Drawing for the job (mm, zero at the part's lowest x, y, z). Coordinates: 2 decimals unless noted, no trailing zeros. Order: outer loops, then holes, each group sorted by start corner. A loop starts at its lowest first (then second) coordinate and runs counter-clockwise, first axis right, second up. Notation, with made-up numbers: (-38.5, -11) -> (-6.5, -11) arc R20 ccw to (-6.5, 18) -> close; hole circle Ø6 at (19, 71.5). An arc over 180 degrees is marked (long way). Write each question's results on one line, items separated by ' | '.
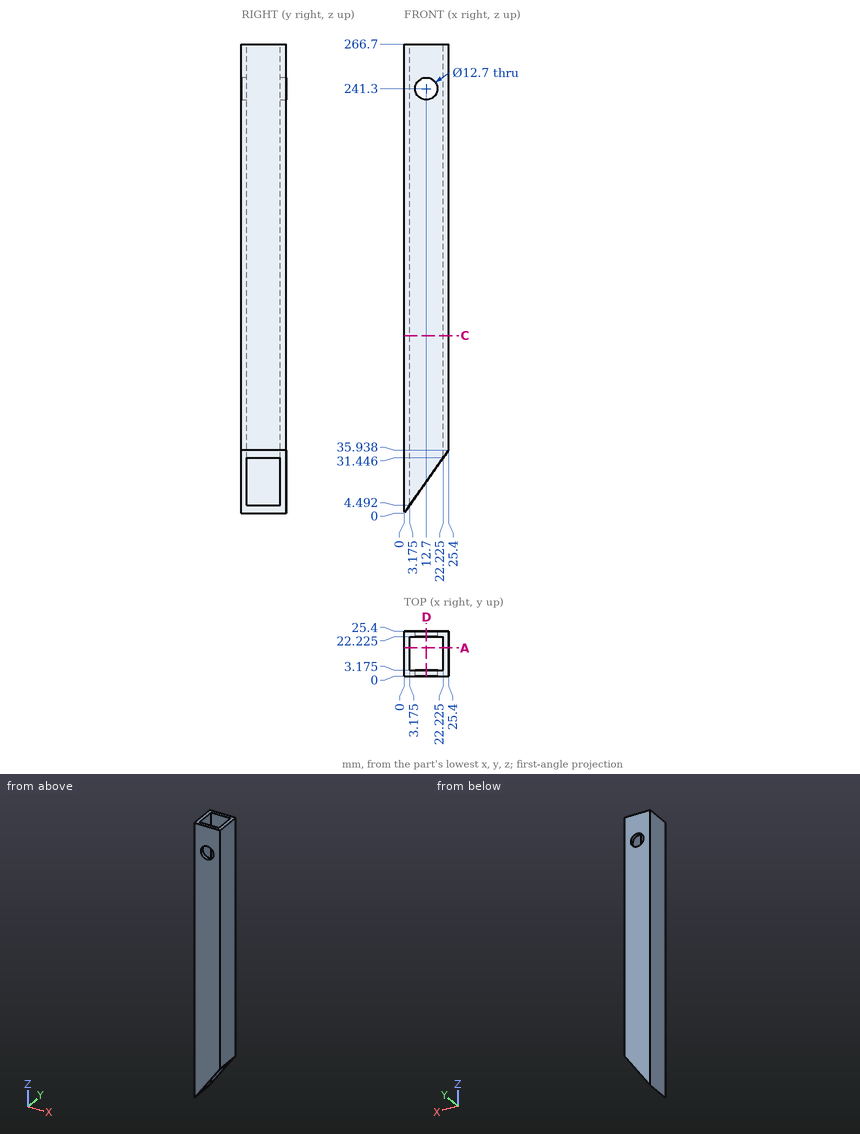
Item 1: Slice it at D-D, the plane x = 12.7. State how many separate pieces and enclosed holes the cut face has, and give its area (3 significant figures).
Answer:
separate pieces: 4 | enclosed holes: 0 | area: 1,500 mm^2
Item 2: Slice it at A-A, the plane y = 16. List the corners of the cut face in (x, z) (1 decimal), and give its area (3 significant figures).
Answer:
outline: (0, 0) -> (3.2, 4.5) -> (3.2, 266.7) -> (0, 266.7) -> close; (22.2, 31.4) -> (25.4, 35.9) -> (25.4, 266.7) -> (22.2, 266.7) -> close | area: 1,580 mm^2
Item 3: Slice it at C-C, the plane z = 101. List the corners of the cut face in (x, y) (1 decimal).
Answer:
outline: (0, 0) -> (25.4, 0) -> (25.4, 25.4) -> (0, 25.4) -> close; hole (3.2, 3.2) -> (22.2, 3.2) -> (22.2, 22.2) -> (3.2, 22.2) -> close
Item 4: Pin check, flat tips, straight feed: pin 1 (2 mm diameter, centred on x = 9.5, z = 238.5, fed in from +Y); pin 2 (8 mm diameter, centred on y = 7.5, z = 28, fed in from +X). Stop position of each tip, or through.
Answer:
pin 1: passes through | pin 2: stops at x = 22.62
Item 5: Drill centre lines: line 1 (Y direction, x = 12.5, z = 92) (1 decimal); line 2 (X direction, y = 24.7, z = 241.3). Where is each one in solid material? Low to high. Write a range as from..to.
Answer:
line 1: y = 0..3.2, 22.2..25.4 | line 2: x = 0..6.35, 19.05..25.4
